Design review of the part shown in the three views and the two pictorial views. Dimensions are in mm from the part's minimum x, y and z. A direction names the side the tool comes from. Coordinates: 2 decimals unless noted, no trailing zeros. Loops run counter-clockwise (first coordinate to the right, second up) from the corner with the lowest first, then second, coordinate; pieces in that order, holes last. Notation, with made-up numbers: M 67,30 L 78,30 A17 cw 78,50 Z; hole C 85.25,22 d8. An arc over 180 degrees is marked long. Use one line per item in the form item = value.
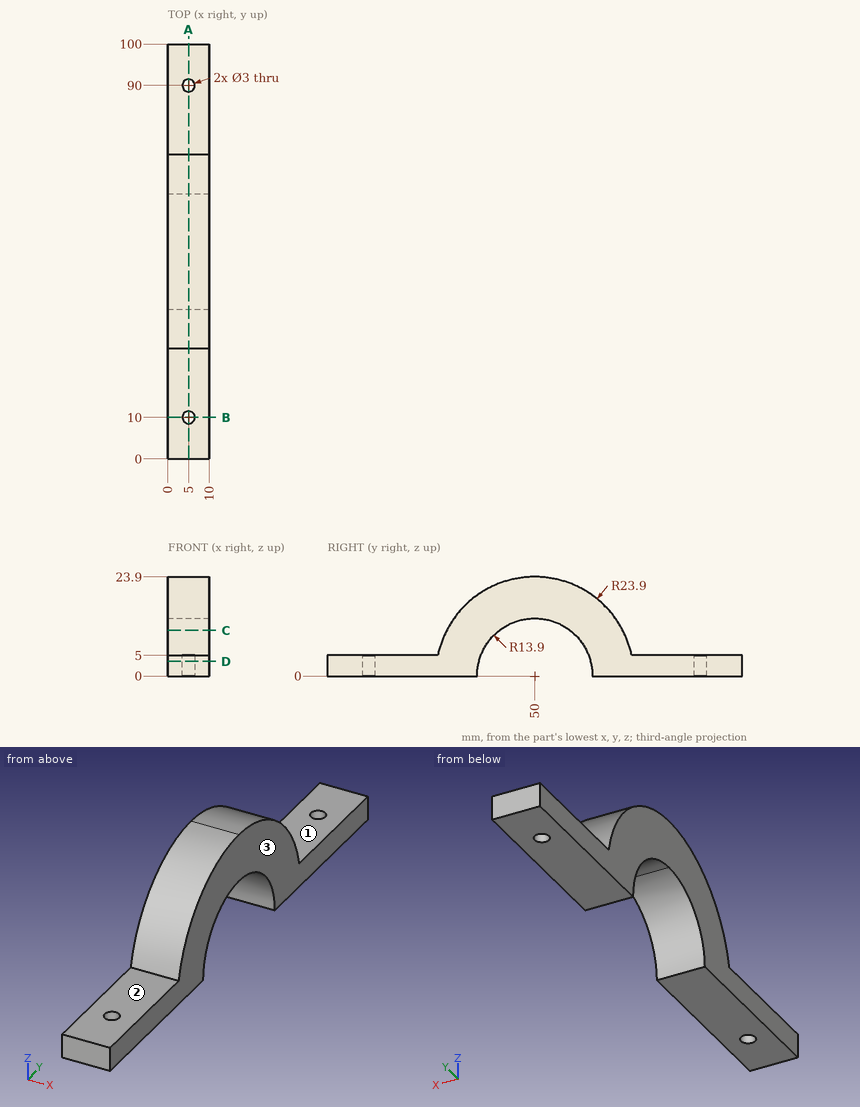
1. Machinability: for the marked faces 1, 2 and 3, which of the approach directions +Z, -Z, +X, -X, +Y, -Y give a long, thin tool a straight path to every point of the face, cutting with its end or side? Answer none if there is none.
Response values:
face_1 = +Z, +X, -X, +Y
face_2 = +Z, +X, -X, -Y
face_3 = +Z, -Z, +X, +Y, -Y
2. Wall thickness on line 1 along X through (y, z) = (90, 1.1); line 2 along Y through (x, z) = (5, 1.2); line 3 along Y through (x, z) = (5, 3.3): over which ranges is each line inside the solid? List them lowest first. Write a range as from..to.
Response values:
line_1 = 0..3.5, 6.5..10
line_2 = 0..8.5, 11.5..36.15, 63.85..88.5, 91.5..100
line_3 = 0..8.5, 11.5..36.5, 63.5..88.5, 91.5..100
3. Add section A-A (x = 5). State the section outline as (y, z) points, then the cut area to 3 significant figures.
Response values:
outline = M 0,0 L 8.5,0 L 8.5,5 L 0,5 Z; M 11.5,0 L 36.1,0 A13.9 cw 50,13.9 A13.9 cw 63.9,0 L 88.5,0 L 88.5,5 L 73.37,5 A23.9 ccw 50,23.9 A23.9 ccw 26.63,5 L 11.5,5 Z; M 91.5,0 L 100,0 L 100,5 L 91.5,5 Z
area = 827 mm^2
4. Add section C-C (z = 11). State the section outline as (x, y) points.
Response values:
outline = M 0,28.78 L 10,28.78 L 10,41.5 L 0,41.5 Z; M 0,58.5 L 10,58.5 L 10,71.22 L 0,71.22 Z
5. Add section B-B (y = 10). State the section outline as (x, z) points.
Response values:
outline = M 0,0 L 3.5,0 L 3.5,5 L 0,5 Z; M 6.5,0 L 10,0 L 10,5 L 6.5,5 Z
6. Insertion check: P1, Ø4, axis at x = 5, y = 90, coming from the +Z side; P2, Ø5, axis at x = 7, z = 15.5, coming from the -Y side; P3, Ø1, axis at x = 3, y = 46, coming from the -Z side. Each pin has a flat end and moves straight along its axis. Give the tip position at first contact, or say it passes through.
Response values:
P1 = 5
P2 = 29.94
P3 = 13.15
7. Add section D-D (z = 3.5). State the section outline as (x, y) points, then the cut area to 3 significant figures.
Response values:
outline = M 0,0 L 10,0 L 10,36.55 L 0,36.55 Z; M 0,63.45 L 10,63.45 L 10,100 L 0,100 Z; hole C 5,10 d3; hole C 5,90 d3
area = 717 mm^2
